Could you check a few things on this model? Use its own coordinates, in mm. Coordinates: 2 decimals unless noted, no trailing zeros. Write each loop counter-clockwise with the first axis right and the second up, starting at its lowest first coordinate (ties: lowest second). Pieces come first, ordered by that corner, then holes.
```python
from build123d import *

# Parameters (mm, degrees)
SKETCH1_R               = 2.4585
BASENUT_DEPTH           = 5.2
ENDCHAMFER_SIZE         = 0.5415
ENDCHAMFER_SIZE2        = 0.312635171
ENDCHAMFER_PART_2_SIZE  = 0.5415
ENDCHAMFER_PART_2_SIZE2 = 0.312635171


with BuildPart() as part:
    # Sketch1 → BaseNut (new body)
    with BuildSketch(Plane.XY):
        Polygon((5.773502692, 0), (2.886751346, 5), (-2.886751346, 5), (-5.773502692, 0), (-2.886751346, -5), (2.886751346, -5), align=None)
        Circle(SKETCH1_R, mode=Mode.SUBTRACT)
    extrude(amount=-BASENUT_DEPTH)

    # Sketch2 → Double-Chamfer (revolve, cut)
    with BuildSketch(Plane(origin=(0, 0, 0), x_dir=(1, 0, 0), z_dir=(0, 1, 0))):
        Polygon((-5.773502692, 5.2), (-4.625, 5.2), (-5.773502692, 4.536911662), align=None)
        Polygon((-5.773502692, 0.663088338), (-5.773502692, 0), (-4.625, 0), align=None)
    revolve(axis=Axis((0, 0, -3.375940562), (0, 0, 1)), mode=Mode.SUBTRACT)

    # EndChamfer
    endchamfer_edges = [part.edges().sort_by_distance(p)[0] for p in [
        (-2.4585, 0, -5.2),
    ]]
    endchamfer_side = [part.faces().sort_by_distance(p)[0] for p in [
        (-2.4585, 0, -2.6),
    ]]
    chamfer(endchamfer_edges, length=ENDCHAMFER_SIZE, length2=ENDCHAMFER_SIZE2, reference=endchamfer_side[0])

    # EndChamfer part 2
    endchamfer_part_2_edges = [part.edges().sort_by_distance(p)[0] for p in [
        (-2.4585, 0, 0),
    ]]
    endchamfer_part_2_side = [part.faces().sort_by_distance(p)[0] for p in [
        (4.494185245, 0, 0),
    ]]
    chamfer(endchamfer_part_2_edges, length=ENDCHAMFER_PART_2_SIZE, length2=ENDCHAMFER_PART_2_SIZE2, reference=endchamfer_part_2_side[0])


solid = part.part
```
1. I want a section at C-C on z = -4.8. Please give me the cut outline in (x, y), plus the area to 3 significant figures.
Verdict:
outline: (-5.24, -0.93) - (-3.42, -4.07) arc R5.32 ccw to (-1.81, -5) - (1.81, -5) arc R5.32 ccw to (3.42, -4.07) - (5.24, -0.93) arc R5.32 ccw to (5.24, 0.93) - (3.42, 4.07) arc R5.32 ccw to (1.81, 5) - (-1.81, 5) arc R5.32 ccw to (-3.42, 4.07) - (-5.24, 0.93) arc R5.32 ccw to start; hole circle Ø5.08 at (0, 0)
area: 63.9 mm2
2. Please list where these lines run through material, in increasing order: line 1 along Y through (x, z) = (0, -2.5); line 2 along X through (y, z) = (-0.75, -1.85); line 3 along X through (y, z) = (1.25, -0.4).
Verdict:
line 1: y = -5 to -2.46, 2.46 to 5
line 2: x = -5.34 to -2.34, 2.34 to 5.34
line 3: x = -5.05 to -2.12, 2.12 to 5.05
3. I want a section at A-A on x = 0. Please give me the cut outline in (y, z) (1 decimal), plus the area to 3 significant figures.
Verdict:
outline: (-5, -5) - (-4.6, -5.2) - (-2.8, -5.2) - (-2.5, -4.7) - (-2.5, -0.3) - (-3, 0) - (-4.6, 0) - (-5, -0.2) - close; (2.5, -4.7) - (2.8, -5.2) - (4.6, -5.2) - (5, -5) - (5, -0.2) - (4.6, 0) - (3, 0) - (2.5, -0.3) - close
area: 25.9 mm2
4. For pin 1 (2 mm diameter, centred on y = -3.5, z = -2.5, fed in from +X); pin 2 (3 mm diameter, centred on x = -4, z = -2.5, fed in from -Y), each with a flat end and sliding along its axis, tell me the tip position at first contact or that it passes through.
Verdict:
pin 1: stops at x = 4.33
pin 2: stops at y = -5
5. If we mould it in two halves opening along X, with no side actions, what happens to faces 1 (the face through (4.31, -2.535, -2.567)), 2 (the face through (-4.31, 2.535, -2.567)), 3 (the face through (2.345, 0.738, -2.455))? For each: pulls with the +X half, pulls with the -X half, needs draft (parallel to the pull), parting line crosses it, or undercut.
Verdict:
face 1: pulls with the +X half
face 2: pulls with the -X half
face 3: undercut
6. I want a section at B-B on z = -2.1. Please give me the cut outline in (x, y), plus the area to 3 significant figures.
Verdict:
outline: (-5.77, 0) - (-2.89, -5) - (2.89, -5) - (5.77, 0) - (2.89, 5) - (-2.89, 5) - close; hole circle Ø4.92 at (0, 0)
area: 67.6 mm2
